Model file for the job. Use its own axes, mm. A direction names the side the tool comes from. Round coordinates to 2 decimals unless told otherwise and drop trailing zeros. Loops run counter-clockwise (first coordinate to the right, second up) from the corner with the lowest first, then second, coordinate; pieces in that order, holes last.
from build123d import *

# Parameters (mm, degrees)
SKETCH1_W                = 95
SKETCH1_H                = 80
SKETCH1_R                = 28
BOSS_EXTRUDE1_DEPTH      = 10
F_5_0_5_DIAMETER_HOLE1_D = 5
SKETCH4_W                = 95
SKETCH4_H                = 18
BOSS_EXTRUDE2_DEPTH      = 10
SKETCH6_W                = 20
SKETCH6_H                = 14
BOSS_EXTRUDE3_DEPTH      = 40
SKETCH10_W               = 50
SKETCH10_H               = 14
BOSS_EXTRUDE4_DEPTH      = 20
SKETCH9_W                = 6.5
SKETCH9_H                = 14.5
CUT_EXTRUDE1_DEPTH       = 20
BOSS_EXTRUDE5_DEPTH      = 5
FILLET3_SIZE             = 10
FILLET3_SIZE_2           = 30
SKETCH15_W               = 10
SKETCH15_H               = 98
CUT_EXTRUDE2_DEPTH       = 6
SKETCH16_W               = 9
SKETCH16_H               = 98
BOSS_EXTRUDE7_DEPTH      = 33
BOSS_EXTRUDE8_DEPTH      = 26.5
CUT_EXTRUDE3_DEPTH       = 6.5
FILLET4_R                = 10
BOSS_EXTRUDE9_DEPTH      = 8.5
FILLET5_R                = 5
FILLET6_R                = 10
CUT_EXTRUDE4_DEPTH       = 133.445770086
CUT_EXTRUDE4_DEPTH_BACK  = 133.445770086
SKETCH20_W               = 6.5
SKETCH20_H               = 14.5


with BuildPart() as part:
    # Sketch1 → Boss-Extrude1 (new body)
    with BuildSketch(Plane(origin=(0, 0, 0), x_dir=(0, 0, -1), z_dir=(1, 0, 0))):
        Rectangle(SKETCH1_W, SKETCH1_H)
        Circle(SKETCH1_R, mode=Mode.SUBTRACT)
    extrude(amount=BOSS_EXTRUDE1_DEPTH)

    # Ø5.0 (5) Diameter Hole1 (through all)
    with Locations(Plane(origin=(10, 0, 0), x_dir=(0, 0, -1), z_dir=(1, 0, 0))):
        with Locations((-32.5, 0), (0, 32.5), (32.5, 0), (0, -32.5)):
            Hole(F_5_0_5_DIAMETER_HOLE1_D / 2)

    # Sketch4 → Boss-Extrude2 (add)
    with BuildSketch(Plane(origin=(10, 0, 0), x_dir=(0, 0, -1), z_dir=(1, 0, 0))):
        with Locations((0, -49)):
            Rectangle(SKETCH4_W, SKETCH4_H)
    extrude(amount=-BOSS_EXTRUDE2_DEPTH)

    # Sketch6 → Boss-Extrude3 (add)
    with BuildSketch(Plane(origin=(10, 0, 0), x_dir=(0, 0, -1), z_dir=(1, 0, 0))):
        with Locations((-37.5, -51)):
            Rectangle(SKETCH6_W, SKETCH6_H)
    extrude(amount=BOSS_EXTRUDE3_DEPTH)

    # Sketch10 → Boss-Extrude4 (add)
    with BuildSketch(Plane.XY.offset(47.5)):
        with Locations((25, -51)):
            Rectangle(SKETCH10_W, SKETCH10_H)
    extrude(amount=BOSS_EXTRUDE4_DEPTH)

    # Sketch9 → Cut-Extrude1 (cut)
    with BuildSketch(Plane(origin=(0, -44, 0), x_dir=(1, 0, 0), z_dir=(0, 1, 0))):
        with Locations((41.75, -50.25)):
            Rectangle(SKETCH9_W, SKETCH9_H)
    extrude(amount=-CUT_EXTRUDE1_DEPTH, mode=Mode.SUBTRACT)

    # Sketch13 → Boss-Extrude5 (add, symmetric)
    with BuildSketch(Plane(origin=(5, 0, 0), x_dir=(0, 0, -1), z_dir=(1, 0, 0))):
        Polygon((-47.5, 40), (-67.5, -44), (-47.5, -44), align=None)
    extrude(amount=BOSS_EXTRUDE5_DEPTH, both=True)

    # Fillet3
    # an asymmetric fillet: 30, 10 mm, written as the material it adds along each edge
    with BuildSketch(Plane(origin=(10, -44, 67.5), x_dir=(1, 0, 0), z_dir=(0, 0, -1))) as fillet3_piece_1_section:
        with BuildLine():
            Bezier((FILLET3_SIZE, 0), (0, 0), (0, -FILLET3_SIZE_2), weights=[1, 0.707106781, 1])
            Line((0, -FILLET3_SIZE_2), (0, 0))
            Line((0, 0), (FILLET3_SIZE, 0))
        make_face()
    fillet3_piece_1 = extrude(amount=40, mode=Mode.PRIVATE)
    fillet3_piece_1 = split(fillet3_piece_1, bisect_by=Plane(origin=(11.956136852, -32.150515723, 64.67869422), z_dir=(0, -0.23162052730603974, -0.9728062146853669)), keep=Keep.TOP, mode=Mode.PRIVATE)
    add(fillet3_piece_1)

    # Sketch15 → Cut-Extrude2 (cut)
    with BuildSketch(Plane(origin=(0, 0, -47.5), x_dir=(-1, 0, 0), z_dir=(0, 0, -1))):
        with Locations((-5, -9)):
            Rectangle(SKETCH15_W, SKETCH15_H)
    extrude(amount=-CUT_EXTRUDE2_DEPTH, mode=Mode.SUBTRACT)

    # Sketch16 → Boss-Extrude7 (add)
    with BuildSketch(Plane(origin=(0, 0, -41.5), x_dir=(-1, 0, 0), z_dir=(0, 0, -1))):
        with Locations((-5.5, -9)):
            Rectangle(SKETCH16_W, SKETCH16_H)
    extrude(amount=BOSS_EXTRUDE7_DEPTH)

    # Sketch17 → Boss-Extrude8 (add)
    with BuildSketch(Plane(origin=(10, 0, 0), x_dir=(0, 0, -1), z_dir=(1, 0, 0))):
        Polygon((50.627369684, 3.19117124), (74.5, 28.786044199), (74.5, -6.213955801), (50.627369684, -31.80882876), align=None)
    extrude(amount=BOSS_EXTRUDE8_DEPTH)

    # Sketch18 → Cut-Extrude3 (cut)
    with BuildSketch(Plane(origin=(36.5, 0, 0), x_dir=(0, 0, -1), z_dir=(1, 0, 0))):
        Polygon((53.696707867, 6.481940621), (61.009528713, -0.338810898), (70.899618415, 10.264779328), (63.58679757, 17.085530846), align=None)
    extrude(amount=-CUT_EXTRUDE3_DEPTH, mode=Mode.SUBTRACT)

    # Fillet4
    fillet4_edges = [part.edges().sort_by_distance(p)[0] for p in [
        (10, 15.98860772, -62.563684842),
        (10, -14.30882876, -50.627369684),
        (10, -19.01139228, -62.563684842),
    ]]
    fillet(fillet4_edges, radius=FILLET4_R)

    # Sketch19 → Boss-Extrude9 (add)
    with BuildSketch(Plane.XZ.offset(58)):
        Polygon((50, 27.5), (10, -23.5), (10, 27.5), align=None)
    extrude(amount=-BOSS_EXTRUDE9_DEPTH)

    # Fillet5
    fillet5_edges = [part.edges().sort_by_distance(p)[0] for p in [
        (35, -44, 27.5),
    ]]
    fillet(fillet5_edges, radius=FILLET5_R)

    # Fillet6
    fillet6_edges = [part.edges().sort_by_distance(p)[0] for p in [
        (10, -49.5, 2),
    ]]
    fillet(fillet6_edges, radius=FILLET6_R)

    # Sketch20 → Cut-Extrude4 (cut, two sides: drawn at the far end of the back side and taken through both)
    with BuildSketch(Plane(origin=(0, -30.588526305, -32.795273685), x_dir=(1, 0, 0), z_dir=(0, 0.6820751518904317, 0.731282084543061)).offset(-CUT_EXTRUDE4_DEPTH_BACK)):
        with Locations((33.25, 48.615317224)):
            Rectangle(SKETCH20_W, SKETCH20_H)
    extrude(amount=CUT_EXTRUDE4_DEPTH + CUT_EXTRUDE4_DEPTH_BACK, mode=Mode.SUBTRACT)


solid = part.part
Q1. Pull direction X, two halves, no side cores. Call faces 1 (the face through (5.42, -1.41, 57.36)), 2 (the face through (36.5, -12, -56)), 3 (the face through (45, -51, 50)): pulls with the +X half, pulls with the -X half, needs draft (parallel to the pull), parting line crosses it, or undercut.
Q2. Tool access for faces 4 (the face through (42, -51, 43)), 5 (the face through (29, -49.5, 17)), 6 (the face through (1, -10, -58)), 7 (the face through (30, 3, -67)): list every direction of +Z, -Z, +X, -X, +Y, -Y with a clear straight run to the whole face (end or side of a thin tool).
Q3. Slice it at D-D on x = 42.5. Give the cut face in (y, z), plus the area to 3 significant figures.
Q4. Probe line 1 (Z direction, x = 5, y = 1); line 2 (Z direction, x = 4, y = -19); line 3 (Y direction, x = 3.5, z = 32.5). List the from-to ranges inside material, lowest first.
Q5. Flat gauge pins, fed straight in: P1, Ø13, axis at x = 28.5, y = -5.5, coming from the +Z side; P2, Ø23, axis at y = -3, z = -66, coming from the +X side; P3, Ø12, axis at y = -8, z = -32, coming from the +X side; P4, Ø6, axis at y = -27.5, z = -16.5, coming from the -X side. Where does each tip first touch, or does it go through?
Q6. Slice it at B-B on x = 4.5. Give the cut face in (y, z).
Q7. Slice it at A-A on z = -18. Give the cut face in (x, y).
Q8. Slice it at C-C on z = 0. Give the cut face in (x, y).
Reply:
1. face 1: needs draft
1. face 2: pulls with the +X half
1. face 3: undercut
2. face 4: +Y, -Y
2. face 5: -Z, +X, +Y
2. face 6: -Z, -X, +Y, -Y
2. face 7: +X
3. outline: (-58, 17.94) - (-49.5, 17.94) - (-49.5, 27.5) - (-49, 27.5) arc R5 ccw to (-44, 32.5) - (-44, 43) - (-58, 43) - close; (-58, 57.5) - (-44, 57.5) - (-44, 67.5) - (-58, 67.5) - close
3. area: 433 mm2
4. line 1: z = -74.5 to -34.79, -30.21 to -27.98, 27.98 to 30.21, 34.79 to 56.79
4. line 2: z = -74.5 to -20.57, 20.57 to 61.55
4. line 3: y = -58 to -2.5, 2.5 to 40
5. P1: stops at z = -50.63
5. P2: stops at x = 36.5
5. P3: stops at x = 10
5. P4: stops at x = 0
6. outline: (-58, -74.5) - (40, -74.5) - (40, 47.5) - (-44, 67.5) - (-58, 67.5) - close; hole circle Ø5 at (-32.5, 0); hole circle Ø56 at (0, 0); hole circle Ø5 at (0, -32.5); hole circle Ø5 at (0, 32.5); hole circle Ø5 at (32.5, 0)
7. outline: (0, -58) - (14.31, -58) - (14.31, -47.73) arc R10 cw to (10, -39.5) - (10, -21.45) - (0, -21.45) - close; (0, 21.45) - (10, 21.45) - (10, 40) - (0, 40) - close
8. outline: (0, -58) - (28.43, -58) - (28.43, -49.5) - (20, -49.5) arc R10 cw to (10, -39.5) - (10, -35) - (0, -35) - close; (0, -30) - (10, -30) - (10, -28) - (0, -28) - close; (0, 28) - (10, 28) - (10, 30) - (0, 30) - close; (0, 35) - (10, 35) - (10, 40) - (0, 40) - close
